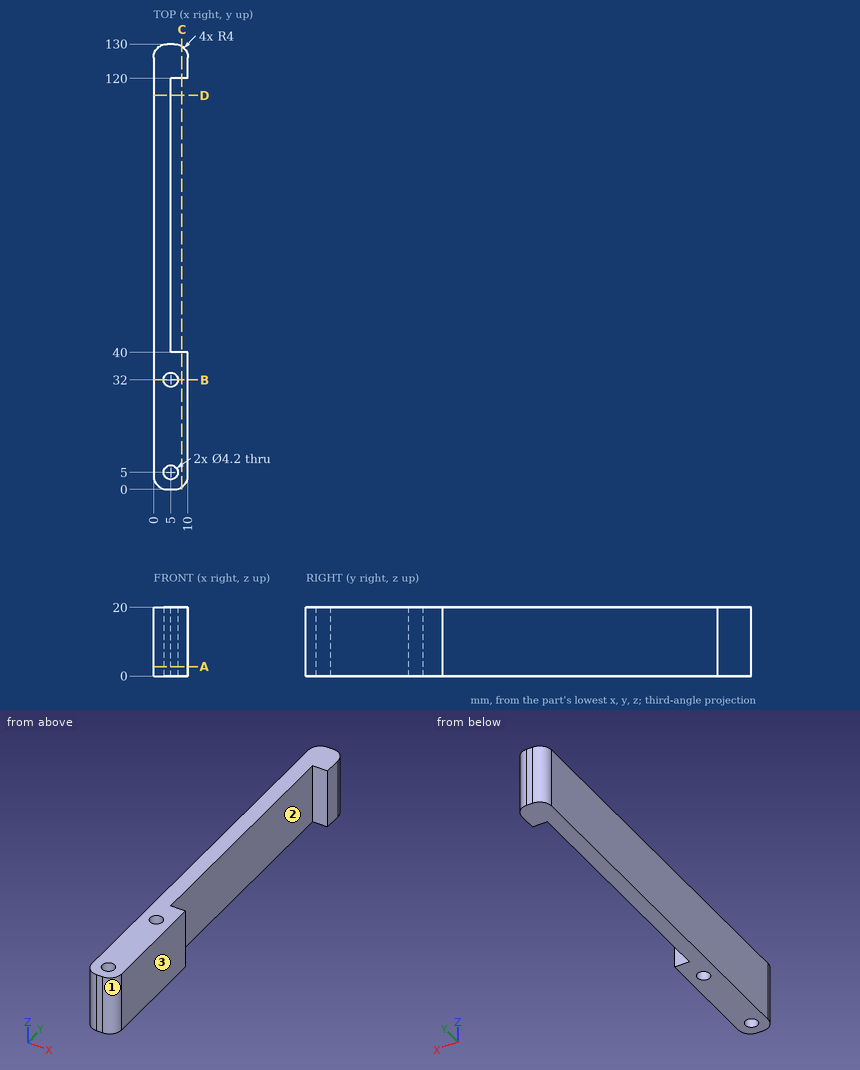
Study the drawing (mm; zero at the part's minimum x, y, z) and answer. Round coordinates to 2 decimals unless told otherwise and drop trailing zeros. Write each loop counter-clockwise with the first axis right and the second up, starting at its lowest first coordinate (ties: lowest second). Pieces come first, ordered by that corner, then holes. Notation, with made-up numbers: (-35.75, 6.5) - (-18.75, 6.5) arc R8 ccw to (-18.75, 13.5) - close; hole circle Ø11 at (3, 43.25). An arc over 180 degrees is marked (long way). Use a Markdown table: item, result. Add a question column.
1. Flat-ended cylindrical pins translate along their axes: P1, Ø1, axis at x = 3, z = 17.5, coming from the -Y side; P2, Ø1, axis at y = 54.5, z = 16, coming from the +X side. Find the tip coordinate at first contact, or state that the pin passes through.
2. The part is cut by section C-C (x = 8.25). Write down the section's boundary in (y, z).
3. For a pull along Y with two mould halves and no side action, classify the marked faces 1, 2 and 3 as +Y half, -Y half, draft (parallel to the pull), parting line (faces both ways), or undercut.
4. Consider line 1 (X direction, y = 5, z = 9.75); line 2 (X direction, y = 110.5, z = 11.75); line 3 (Y direction, x = 4, z = 8.25). Determine where each line is inside the solid, lowest interval first.
5. The part is cut by section B-B (y = 32). Write down the section's boundary in (x, z).
6. The part is cut by section D-D (y = 115). Write down the section's boundary in (x, z), and give its area (3 significant figures).
7. The part is cut by section A-A (z = 2.75). Write down the section's boundary in (x, y).
Reported:
| question | item | result |
|---|---|---|
| 1 | P1 | y = 0.03 |
| 1 | P2 | x = 5 |
| 2 | outline | (0.69, 0) - (40, 0) - (40, 20) - (0.69, 20) - close; (120, 0) - (129.31, 0) - (129.31, 20) - (120, 20) - close |
| 3 | face 1 | -Y half |
| 3 | face 2 | undercut |
| 3 | face 3 | draft |
| 4 | line 1 | 0 to 2.9, 7.1 to 10 |
| 4 | line 2 | 0 to 5 |
| 4 | line 3 | 0 to 3.15, 6.85 to 30.15, 33.85 to 130 |
| 5 | outline | (0, 0) - (2.9, 0) - (2.9, 20) - (0, 20) - close; (7.1, 0) - (10, 0) - (10, 20) - (7.1, 20) - close |
| 6 | outline | (0, 0) - (5, 0) - (5, 20) - (0, 20) - close |
| 6 | area | 100 mm^2 |
| 7 | outline | (0, 4) arc R4 ccw to (4, 0) - (6, 0) arc R4 ccw to (10, 4) - (10, 40) - (5, 40) - (5, 120) - (10, 120) - (10, 126) arc R4 ccw to (6, 130) - (4, 130) arc R4 ccw to (0, 126) - close; hole circle Ø4.2 at (5, 5); hole circle Ø4.2 at (5, 32) |
